from build123d import *

# Parameters (mm, degrees)
F1_DEPTH = 2.4
F2_DEPTH = 1.6


with BuildPart() as f1:
    # F0 (on Top) → F1 (new body)
    with BuildSketch(Plane.XY):
        with BuildLine():
            ThreePointArc((6.2364408078, 3.1791203265), (5.4557408837, 4.3857600721), (4.4450679147, 5.4075291247))
            ThreePointArc((4.4450679147, 5.4075291247), (4.1248628557, 3.8877917046), (4.4076455939, 2.3606482835))
            ThreePointArc((4.4076455939, 2.3606482835), (4.5207987432, 2.1359725475), (4.6225083364, 1.9058899968))
            Line((4.6225083364, 1.9058899968), (6.3735347613, 2.8722783552))
            ThreePointArc((6.3735347613, 2.8722783552), (6.2985312404, 3.0228146209), (6.2364408078, 3.1791203265))
        make_face()
        with BuildLine():
            ThreePointArc((12.1245611862, 3.8386667137), (8.9251943462, 7.7577210056), (4.4450679147, 5.4075291247))
            ThreePointArc((4.4450679147, 5.4075291247), (5.4557408837, 4.3857600721), (6.2364408078, 3.1791203265))
            ThreePointArc((6.2364408078, 3.1791203265), (7.7900770735, 5.8104984454), (10.1245611862, 3.8386667137))
            ThreePointArc((10.1245611862, 3.8386667137), (9.7517195067, 2.6757583768), (8.7722053863, 1.9464307373))
            Line((8.7722053863, 1.9464307373), (9.4198495864, 0.054194761))
            ThreePointArc((9.4198495864, 0.054194761), (11.3788778273, 1.51285004), (12.1245611862, 3.8386667137))
        make_face()
        with BuildLine():
            ThreePointArc((4.4450679147, 5.4075291247), (-6.3291182404, -2.9903615666), (7, 0))
            ThreePointArc((7, 0), (5.6226632008, 0.717688266), (4.6225083364, 1.9058899968))
            ThreePointArc((4.6225083364, 1.9058899968), (4.9047192418, 0.9714572348), (5, 0))
            ThreePointArc((5, 0), (-4.8496509137, -1.2169166016), (4.4076455939, 2.3606482835))
            ThreePointArc((4.4076455939, 2.3606482835), (4.1248628557, 3.8877917046), (4.4450679147, 5.4075291247))
        make_face()
        with BuildLine():
            ThreePointArc((4.6225083364, 1.9058899968), (5.6226632008, 0.717688266), (7, 0))
            ThreePointArc((7, 0), (6.8524662966, 1.4295823353), (6.416084099, 2.7989042203))
            ThreePointArc((6.416084099, 2.7989042203), (6.3944204178, 2.8353657012), (6.3735347613, 2.8722783552))
            Line((6.3735347613, 2.8722783552), (4.6225083364, 1.9058899968))
        make_face()
    extrude(amount=-F1_DEPTH)

    # F0 (on Top) → F2 (cut)
    with BuildSketch(Plane.XY):
        with BuildLine():
            ThreePointArc((12.1245611862, 3.8386667137), (8.9251943462, 7.7577210056), (4.4450679147, 5.4075291247))
            ThreePointArc((4.4450679147, 5.4075291247), (5.4557408837, 4.3857600721), (6.2364408078, 3.1791203265))
            ThreePointArc((6.2364408078, 3.1791203265), (7.7900770735, 5.8104984454), (10.1245611862, 3.8386667137))
            ThreePointArc((10.1245611862, 3.8386667137), (9.7517195067, 2.6757583768), (8.7722053863, 1.9464307373))
            Line((8.7722053863, 1.9464307373), (9.4198495864, 0.054194761))
            ThreePointArc((9.4198495864, 0.054194761), (11.3788778273, 1.51285004), (12.1245611862, 3.8386667137))
        make_face()
    extrude(amount=-F2_DEPTH, mode=Mode.SUBTRACT)


solid = f1.part
Can you work these out from the model? Positions are in its coordinate system, mm. A direction names the side the tool comes from. Round coordinates to 2 decimals unless told otherwise and drop trailing zeros. Write each loop counter-clockwise with the first axis right and the second up, starting at its lowest first coordinate (ties: lowest second). Pieces come first, ordered by that corner, then holes. Notation, with made-up numbers: (89.5, -38.5) - (95.5, -38.5) arc R5 cw to (95.5, -29.5) - close; hole circle Ø7 at (-0.5, 28). An arc over 180 degrees is marked (long way). Write each question's results on one line, items separated by ' | '. Start each with the question number.
1) Which directions (+Z, -Z, +X, -X, +Y, -Y) give clear straight access to the entire face, cutting with the end or side of a thin tool? Please do faces 1 (the flat face through (9, 6, -1.6)), 2 (the flat face through (5.4, 1, -2.4)).
2) Suppose I cut it at D-D (y = 3.5). List the corners of the cut face in (x, z) for me, and give its area (3 significant figures).
3) Please list where these lines run through material, in increasing order: line 1 (X direction, y = 0, z = -0.75); line 2 (X direction, y = 4.25, z = -1.8); line 3 (Z direction, x = 10.25, y = 4.75).
4) Suppose I cut it at C-C (y = -2.25). List the corners of the cut face in (x, z) for me.
5) Suppose I cut it at A-A (x = 0). List the corners of the cut face in (y, z) for me, and give its area (3 significant figures).
6) Suppose I cut it at B-B (z = -1.1). List the corners of the cut face in (x, y) for me, and give its area (3 significant figures).
7) For pin 1 Ø3.5 at (x, y) = (8.12, 3.84) entering from -Z, with a flat end and sliding along its axis, tell me the tip position at first contact or that it passes through.
Here are the results:
1) face 1: +Z, +X, +Y | face 2: -Z, +X, -X, +Y, -Y
2) outline: (-6.06, -2.4) - (-3.57, -2.4) - (-3.57, 0) - (-6.06, 0) - close; (3.57, -2.4) - (6.15, -2.4) - (6.15, -1.6) - (6.06, -1.6) - (6.06, 0) - (3.57, 0) - close; (10.1, -2.4) - (12.11, -2.4) - (12.11, -1.6) - (10.1, -1.6) - close | area: 13.6 mm2
3) line 1: x = -7 to -5, 5 to 7 | line 2: x = -5.56 to -2.63, 2.63 to 6.17, 10.08 to 12.1 | line 3: z = -2.4 to -1.6
4) outline: (-6.63, -2.4) - (-4.47, -2.4) - (-4.47, 0) - (-6.63, 0) - close; (4.47, -2.4) - (6.63, -2.4) - (6.63, 0) - (4.47, 0) - close
5) outline: (-7, -2.4) - (-5, -2.4) - (-5, 0) - (-7, 0) - close; (5, -2.4) - (7, -2.4) - (7, 0) - (5, 0) - close | area: 9.60 mm2
6) outline: (6.24, 3.18) arc R7 ccw (long way) to (6.42, 2.8) arc R2 cw to start; hole circle Ø10 at (0, 0) | area: 75.4 mm2
7) pin 1: passes through
